Autodesk Inventor part; units mm, degrees
ref_plane "YZ Plane" through (0, 0, 0) normal (1, 0, 0) x (0, 1, 0)
ref_plane "XZ Plane" through (0, 0, 0) normal (0, 1, 0) x (-1, 0, 0)
ref_plane "XY Plane" through (0, 0, 0) normal (0, 0, 1) x (1, 0, 0)
sketch "Sketch1" plane through (0, 0, 0) normal (0, 0, 1) x (1, 0, 0)
  line L0 (0, 0) -> (68, 0)
  line L1 (68, 0) -> (68, 24)
  line L2 (68, 24) -> (0, 24)
  line L3 (0, 24) -> (0, 0)
  dimension "d0" = 68
  dimension "d1" = 24
extrude "Extrusion1" add sketch "Sketch1" along normal blind 2
sketch "Sketch2" plane through (0, 0, 2) normal (0, 0, 1) x (1, 0, 0)
  circle A0 centre (6.2, 16) radius 2.4
  circle A1 centre (61.8, 16) radius 2.4
  line L0 (68, 24) -> (0, 24)
  line L1 (34, 24) -> (34, 0) construction
  line L2 (0, 0) -> (68, 0)
  dimension "d4" = 4.8
  dimension "d5" = 4.8
  dimension "d6" = 55.6
  dimension "d7" = 27.8
  dimension "d8" = 8
extrude "Extrusion2" cut sketch "Sketch2" against normal blind 2
sketch "Sketch3" plane through (0, 0, 0) normal (0, 0, -1) x (-1, 0, 0)
  line L0 (-68, 24) -> (0, 24)
  line L1 (-68, 0) -> (-68, 24)
  line L2 (0, 24) -> (-68, 24)
  line L3 (-68, 24) -> (-68, 22)
  line L4 (-68, 22) -> (0, 22)
  line L5 (0, 22) -> (0, 24)
  point P0 (0, 0)
  dimension "d11" = 2
extrude "Extrusion3" add sketch "Sketch3" along normal blind 38
sketch "Sketch4" plane through (0, 0, 0) normal (0, 0, -1) x (-1, 0, 0)
  line L0 (-68, 0) -> (-68, 24)
  line L1 (-68, 0) -> (0, 0)
  line L2 (0, 0) -> (0, 2)
  line L3 (0, 2) -> (-68, 2)
  line L4 (-68, 2) -> (-68, 0)
  line L5 (0, 22) -> (0, 0)
  dimension "d14" = 2
extrude "Extrusion4" add sketch "Sketch4" along normal blind 10
properties part number "MainsCoverInternal"
Check sheet for the modelled part. Datum: model origin and axes. Units: mm. A direction names the side the tool comes from. Round coordinates to 2 decimals unless told otherwise and drop trailing zeros. Loops run counter-clockwise (first coordinate to the right, second up) from the corner with the lowest first, then second, coordinate; pieces in that order, holes last. Notation, with made-up numbers: M 40,-32 L 80,-32 A18 cw 80,-6 Z; hole C -19.5,-8.75 d7. An arc over 180 degrees is marked long. One line per item, written item: value.
(1) Depth check by flat-ended pin: pin 1 Ø2 at (x, y) = (17.5, 1.5) entering from -Z; pin 2 Ø8 at (x, y) = (17.5, 10.5) entering from -Z; pin 3 Ø4.5 at (x, y) = (6.2, 16) entering from +Z; pin 4 Ø19 at (x, z) = (36.5, -23.5) entering from -Y. Enter the tip coordinate at first touch or a pass-through.
Computed values:
pin 1: stops at z = -10
pin 2: stops at z = 0
pin 3: passes through
pin 4: stops at y = 22
(2) Sectioned sample at D-D, the plane x = 20.5. Record the cut outline in (y, z).
Computed values:
outline: M 0,-10 L 2,-10 L 2,0 L 22,0 L 22,-38 L 24,-38 L 24,2 L 0,2 Z
(3) Sectioned sample at B-B, the plane z = -9. Record the cut outline in (x, y).
Computed values:
outline: M 0,0 L 68,0 L 68,2 L 0,2 Z; M 0,22 L 68,22 L 68,24 L 0,24 Z
(4) Sectioned sample at A-A, the plane x = 6.2. Record the cut outline in (y, z), then the cut area to 3 significant figures.
Computed values:
outline: M 0,-10 L 2,-10 L 2,0 L 13.6,0 L 13.6,2 L 0,2 Z; M 18.4,0 L 22,0 L 22,-38 L 24,-38 L 24,2 L 18.4,2 Z
area: 134 mm^2
(5) Thickness scan on line 1 (Y direction, x = 29, z = -3.5); line 2 (Y direction, x = 6, z = 1); line 3 (Z direction, x = 59, y = 1.5). Record the ranges inside material, lowest first.
Computed values:
line 1: y = 0 to 2, 22 to 24
line 2: y = 0 to 13.61, 18.39 to 24
line 3: z = -10 to 2
(6) Access from +Z, -Z, +X, -X, +Y, -Y to the whole of each face (thin tool, end or side, straight path). Record for faces 4 (the face through (68, 23, -10)), 5 (the face through (34, 1, -10)), 6 (the face through (34, 2, -5)).
Computed values:
face 4: +Z, -Z, +X, +Y, -Y
face 5: -Z, +X, -X, -Y
face 6: -Z, +X, -X
(7) Release check for a two-part mould opening along Y. For faces 1 (the face through (34, 22, -19)), 2 (the face through (34, 23, -38)), 3 (the face through (34, 24, -18)) record: +Y half, -Y half, draft (parallel to the pull), parting line (faces both ways), or undercut.
Computed values:
face 1: undercut
face 2: draft
face 3: +Y half
(8) Sectioned sample at C-C, the plane y = 16. Record the cut outline in (x, z), then the cut area to 3 significant figures.
Computed values:
outline: M 0,0 L 3.8,0 L 3.8,2 L 0,2 Z; M 8.6,0 L 59.4,0 L 59.4,2 L 8.6,2 Z; M 64.2,0 L 68,0 L 68,2 L 64.2,2 Z
area: 117 mm^2
